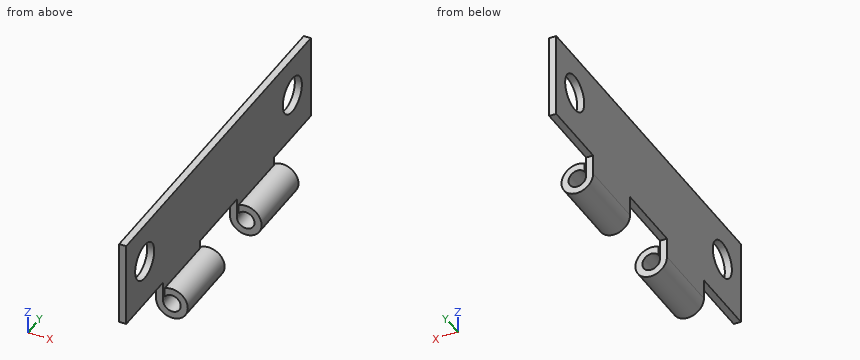
```python
from build123d import *

# Parameters (mm, degrees)
BOSS_EXTRUDE2_DEPTH = 31.75
SKETCH8_W           = 3.6195
SKETCH8_H           = 6.35
CUT_EXTRUDE3_DEPTH  = 3.8575
SKETCH15_R          = 1.6383
CUT_EXTRUDE5_DEPTH  = 3.8575


with BuildPart() as part:
    # Sketch4 → Boss-Extrude2 (new body)
    with BuildSketch(Plane(origin=(0, 0, 0), x_dir=(1, 0, 0), z_dir=(0, 1, 0))):
        with BuildLine():
            Line((0, 0), (0, -9.525))
            Line((0, -9.525), (0.635, -9.525))
            Line((0.635, -9.525), (0.635, 0))
            ThreePointArc((0.635, 0), (2.190088254, 0.224506403), (0.762, -0.430677954))
            Line((0.762, -0.430677954), (0.762, -1.263634045))
            ThreePointArc((0.762, -1.263634045), (2.652258403, 0.737803327), (0, 0))
        make_face()
    extrude(amount=BOSS_EXTRUDE2_DEPTH)

    # Sketch8 → Cut-Extrude3 (cut, through all)
    with BuildSketch(Plane(origin=(0, 0, 0), x_dir=(0, 0, -1), z_dir=(1, 0, 0))):
        with Locations((0, 3.175)):
            Rectangle(SKETCH8_W, SKETCH8_H)
        with Locations((0, 15.875)):
            Rectangle(SKETCH8_W, SKETCH8_H)
        with Locations((0, 28.575)):
            Rectangle(SKETCH8_W, SKETCH8_H)
    extrude(amount=CUT_EXTRUDE3_DEPTH, mode=Mode.SUBTRACT)

    # Sketch15 → Cut-Extrude5 (cut, through all)
    with BuildSketch(Plane(origin=(0, 0, 0), x_dir=(0, 0, -1), z_dir=(1, 0, 0))):
        with Locations((-5.9436, 3.175)):
            Circle(SKETCH15_R)
    cut_extrude5 = extrude(amount=CUT_EXTRUDE5_DEPTH, mode=Mode.SUBTRACT)

    # Mirror1: Cut-Extrude5 across plane
    add(cut_extrude5.mirror(Plane(origin=(0, 15.875, 0), x_dir=(0, 0, 1), z_dir=(0, -1, 0))), mode=Mode.SUBTRACT)


solid = part.part
```
Part model, mm, in its own coordinate system. Round coordinates to 2 decimals unless told otherwise and drop trailing zeros. Loops run counter-clockwise (first coordinate to the right, second up) from the corner with the lowest first, then second, coordinate; pieces in that order, holes last. Notation, with made-up numbers: (-10, -31) -> (28, -31) arc R17 cw to (28, -8) -> close; hole circle Ø3 at (87, -11). An arc over 180 degrees is marked (long way). Use a Markdown table: item, result.
1) Cut at D-D, the plane y = 9. List the corners of the cut face in (x, z) (1 decimal).
The answers:
| item | result |
|---|---|
| outline | (0, 0) arc R1.4 ccw (long way) to (0.8, 1.3) -> (0.8, 0.4) arc R0.8 cw (long way) to (0.6, 0) -> (0.6, 9.5) -> (0, 9.5) -> close |
2) Probe line 1 (Y direction, x = 0.45, z = 0); line 2 (X direction, y = 16, z = 2.25) (3 decimals); line 3 (Z direction, x = 2.05, y = 19.5). List the from-to ranges inside material, lowest first. Write a range as [from, to].
The answers:
| item | result |
|---|---|
| line 1 | y = [6.35, 12.7], [19.05, 25.4] |
| line 2 | x = [0, 0.635] |
| line 3 | z = [-1.29, -0.49], [0.49, 1.29] |
3) Drop flat-ended pins along their axis: pin 1 Ø1.4 at (x, z) = (2, 0) entering from -Y; pin 2 Ø1 at (x, z) = (2, 1) entering from +Y; pin 3 Ø1.5 at (x, y) = (0.5, 26.5) entering from -Z. Give the stop position or say it passes through.
The answers:
| item | result |
|---|---|
| pin 1 | stops at y = 6.35 |
| pin 2 | stops at y = 25.4 |
| pin 3 | stops at z = 1.81 |
4) Cut at A-A, the plane x = 1.4. List the corners of the cut face in (y, z), and give its area (3 significant figures).
The answers:
| item | result |
|---|---|
| outline | (6.35, -1.43) -> (12.7, -1.43) -> (12.7, -0.79) -> (6.35, -0.79) -> close; (6.35, 0.79) -> (12.7, 0.79) -> (12.7, 1.43) -> (6.35, 1.43) -> close; (19.05, -1.43) -> (25.4, -1.43) -> (25.4, -0.79) -> (19.05, -0.79) -> close; (19.05, 0.79) -> (25.4, 0.79) -> (25.4, 1.43) -> (19.05, 1.43) -> close |
| area | 16.1 mm2 |
5) Cut at B-B, the plane z = 6.75. List the corners of the cut face in (x, y) (3 decimals), and give its area (3 significant figures).
The answers:
| item | result |
|---|---|
| outline | (0, 0) -> (0.635, 0) -> (0.635, 1.749) -> (0, 1.749) -> close; (0, 4.601) -> (0.635, 4.601) -> (0.635, 27.149) -> (0, 27.149) -> close; (0, 30.001) -> (0.635, 30.001) -> (0.635, 31.75) -> (0, 31.75) -> close |
| area | 16.5 mm2 |
6) Cut at C-C, the plane y = 3.5. List the corners of the cut face in (x, z) (3 decimals), and give its area (3 significant figures).
The answers:
| item | result |
|---|---|
| outline | (0, 1.81) -> (0.635, 1.81) -> (0.635, 4.338) -> (0, 4.338) -> close; (0, 7.549) -> (0.635, 7.549) -> (0.635, 9.525) -> (0, 9.525) -> close |
| area | 2.86 mm2 |
